Could you check a few things on this model? Use its own coordinates, in mm. Face numbers are marked on the shaded views. A direction names the side the tool comes from. Coordinates: 2 decimals unless noted, no trailing zeros. Loops run counter-clockwise (first coordinate to the right, second up) from the corner with the lowest first, then second, coordinate; pieces in that order, holes last.
1) For the marked faces 1 and 2, which set-ups out of +Z, -Z, +X, -X, +Y, -Y let a thin tool reach every point of the face, with its end or its side?
2) Imagine slicing it at B-B on z = -13.5. Please give me the cut outline in (x, y).
3) Will these pins go through, and if not, where does the flat tip stop? P1, Ø1.5, axis at x = 0, z = -11.5, coming from the +Y side; P2, Ø0.9, axis at x = 0.5, y = 0, coming from the +Z side; P3, Ø5, axis at y = 0, z = -33, coming from the +X side.
4) If I drill on line 1 along Y through (x, z) = (-2, -43); line 2 along Y through (x, z) = (-0.25, -3); line 3 along X through (y, z) = (1.75, -1.5), over which ranges is the centre line in solid material (lowest first)?
5) Imagine slicing it at A-A on x = 0. Please give me the cut outline in (y, z).
```python
from build123d import *

# Parameters (mm, degrees)
CUT_EXTRUDE1_DEPTH = 3.3
CHAMFER1_SIZE      = 0.49075


with BuildPart() as part:
    # Sketch1 → Revolve1 (revolve)
    with BuildSketch(Plane(origin=(0, 0, 0), x_dir=(1, 0, 0), z_dir=(0, 1, 0))):
        Polygon((2.5, 50), (0, 50), (0, 0), (5, 0), (5, 0.3), (2.5, 2.8), align=None)
    revolve(axis=Axis((0, 0, -50), (0, 0, 1)))

    # Sketch2 → Cut-Extrude1 (cut)
    with BuildSketch(Plane.XY):
        Polygon((-0.866025404, -1.5), (0.866025404, -1.5), (1.732050808, 0), (0.866025404, 1.5), (-0.866025404, 1.5), (-1.732050808, 0), align=None)
    extrude(amount=-CUT_EXTRUDE1_DEPTH, mode=Mode.SUBTRACT)

    # Chamfer1
    chamfer1_edges = [part.edges().sort_by_distance(p)[0] for p in [
        (-2.5, 0, -50),
    ]]
    chamfer(chamfer1_edges, length=CHAMFER1_SIZE)


solid = part.part
```
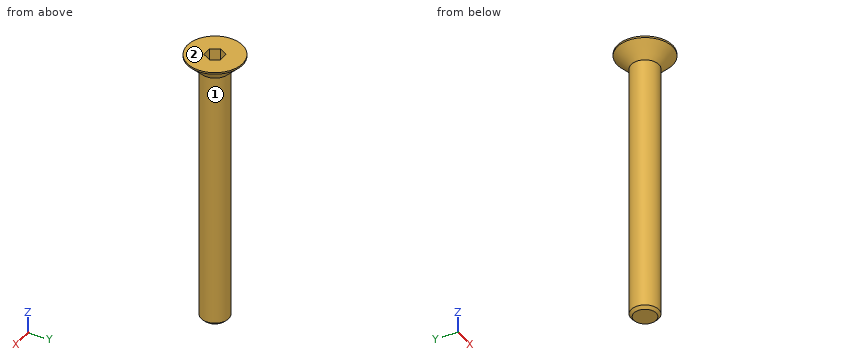
Filled in:
1. face 1: -Z
1. face 2: +Z, +X, -X, +Y, -Y
2. outline: circle Ø5 at (0, 0)
3. P1: stops at y = 2.5
3. P2: stops at z = -3.3
3. P3: stops at x = 2.5
4. line 1: y = -1.5 to 1.5
4. line 2: y = -2.49 to -1.5, 1.5 to 2.49
4. line 3: x = -3.37 to 3.37
5. outline: (-5, -0.3) - (-2.5, -2.8) - (-2.5, -49.51) - (-2.01, -50) - (2.01, -50) - (2.5, -49.51) - (2.5, -2.8) - (5, -0.3) - (5, 0) - (1.5, 0) - (1.5, -3.3) - (-1.5, -3.3) - (-1.5, 0) - (-5, 0) - close
